Could you check a few things on this model? Use its own coordinates, in mm. A direction names the side the tool comes from. Give positions to 0.01 mm unless a question says otherwise; leave off trailing zeros. Write each loop counter-clockwise with the first axis right and the second up, starting at its lowest first coordinate (ties: lowest second). Pieces come first, ordered by that corner, then holes. Notation, with made-up numbers: M -28,-8.75 L -19,-8.75 A28 cw -19,19.25 Z; hole C 12,5 d7. An arc over 180 degrees is marked long. Use one line per item in the form item = value.
from build123d import *

# Parameters (mm, degrees)
CROQUIS1_W              = 45.25
CROQUIS1_H              = 20.4
SALIENTE_EXTRUIR1_DEPTH = 3
CROQUIS2_W              = 10.2
CROQUIS2_H              = 3
CORTAR_EXTRUIR1_DEPTH   = 50.726476851
CORTAR_EXTRUIR2_DEPTH   = 1.05
CROQUIS5_R              = 1.05
CORTAR_EXTRUIR4_DEPTH   = 50.726476851
SALIENTE_EXTRUIR2_DEPTH = 30
CROQUIS8_W              = 45.25
CROQUIS8_H              = 30
CORTAR_EXTRUIR5_DEPTH   = 10
CROQUIS10_R             = 1.65
CORTAR_EXTRUIR6_DEPTH   = 58.197574249
CROQUIS11_W             = 45.25
CROQUIS11_H             = 30
CORTAR_EXTRUIR7_DEPTH   = 2


with BuildPart() as part:
    # Croquis1 → Saliente-Extruir1 (new body)
    with BuildSketch(Plane(origin=(0, 0, 0), x_dir=(1, 0, 0), z_dir=(0, 1, 0))):
        with Locations((22.625, 10.2)):
            Rectangle(CROQUIS1_W, CROQUIS1_H)
    extrude(amount=SALIENTE_EXTRUIR1_DEPTH)

    # Croquis2 → Cortar-Extruir1 (cut, through all)
    with BuildSketch(Plane(origin=(0, 3, 0), x_dir=(1, 0, 0), z_dir=(0, 1, 0))):
        with Locations((22.625, 1.5)):
            Rectangle(CROQUIS2_W, CROQUIS2_H)
    extrude(amount=-CORTAR_EXTRUIR1_DEPTH, mode=Mode.SUBTRACT)

    # Croquis3 → Cortar-Extruir2 (cut)
    with BuildSketch(Plane(origin=(0, 3, 0), x_dir=(1, 0, 0), z_dir=(0, 1, 0))):
        Polygon((42.5, 0), (27.725, 0), (27.725, 4.51852132), (17.525, 4.51852132), (17.525, 0), (2.75, 0), (2.75, 2.75), (0, 2.75), (0, 17.65), (2.75, 17.65), (2.75, 20.4), (42.5, 20.4), (42.5, 17.65), (45.25, 17.65), (45.25, 2.75), (42.5, 2.75), align=None)
    extrude(amount=-CORTAR_EXTRUIR2_DEPTH, mode=Mode.SUBTRACT)

    # Croquis5 → Cortar-Extruir4 (cut, through all)
    with BuildSketch(Plane(origin=(0, 3, 0), x_dir=(1, 0, 0), z_dir=(0, 1, 0))):
        with Locations(Location((43.85, 18.96, 0), (0, 0, 270))):
            Circle(CROQUIS5_R)
        with Locations(Location((1.4, 18.96, 0), (0, 0, 90))):
            Circle(CROQUIS5_R)
        with Locations(Location((43.85, 1.44, 0), (0, 0, 90))):
            Circle(CROQUIS5_R)
        with Locations(Location((1.4, 1.44, 0), (0, 0, 270))):
            Circle(CROQUIS5_R)
    extrude(amount=-CORTAR_EXTRUIR4_DEPTH, mode=Mode.SUBTRACT)

    # Croquis6 → Saliente-Extruir2 (add)
    with BuildSketch(Plane.XZ):
        Polygon((17.525, -3), (0, -3), (0, -18), (45.25, -18), (45.25, -3), align=None)
    extrude(amount=SALIENTE_EXTRUIR2_DEPTH)

    # Croquis8 → Cortar-Extruir5 (cut)
    with BuildSketch(Plane.XY.offset(-3)):
        with Locations((22.625, -15)):
            Rectangle(CROQUIS8_W, CROQUIS8_H)
    extrude(amount=-CORTAR_EXTRUIR5_DEPTH, mode=Mode.SUBTRACT)

    # Croquis10 → Cortar-Extruir6 (cut, through all)
    with BuildSketch(Plane(origin=(0, 0, -18), x_dir=(-1, 0, 0), z_dir=(0, 0, -1))):
        with Locations((-11.3125, -15)):
            Circle(CROQUIS10_R)
        with Locations((-33.9375, -15)):
            Circle(CROQUIS10_R)
    extrude(amount=-CORTAR_EXTRUIR6_DEPTH, mode=Mode.SUBTRACT)

    # Croquis11 → Cortar-Extruir7 (cut)
    with BuildSketch(Plane(origin=(0, 0, -18), x_dir=(-1, 0, 0), z_dir=(0, 0, -1))):
        with Locations((-22.625, -15)):
            Rectangle(CROQUIS11_W, CROQUIS11_H)
    extrude(amount=-CORTAR_EXTRUIR7_DEPTH, mode=Mode.SUBTRACT)


solid = part.part
1) I want a section at B-B, the plane y = -15. Please give me the cut outline in (x, z).
Checked values:
outline = M 0,-16 L 9.66,-16 L 9.66,-13 L 0,-13 Z; M 12.96,-16 L 32.29,-16 L 32.29,-13 L 12.96,-13 Z; M 35.59,-16 L 45.25,-16 L 45.25,-13 L 35.59,-13 Z
2) For faces 5 (the flat face through (22.7, 2.5, -4.519)), 6 (the flat face through (42.5, 2.5, -19)), 7 (the flat face through (27.725, 2.5, -3.7)), which set-ups out of +Z, -Z, +X, -X, +Y, -Y let a thin tool reach every point of the face, with its end or its side?
Checked values:
face_5 = -Z, +X, -X, +Y
face_6 = +Z, -Z, +Y
face_7 = +Z, -Z, +X, +Y
3) Thinking about a two-plate mould opening in Z: for faces 1 (the flat face through (1.4, 2.5, -17.65)), 2 (the flat face through (17.525, 2.5, -3.8)), 3 (the flat face through (22, -15, -13)), 4 (the flat face through (1.4, 2.5, -2.75)), which applies, released by +Z, released by -Z, zero draft, split by the parting line, or undercut?
Checked values:
face_1 = undercut
face_2 = zero draft
face_3 = released by +Z
face_4 = undercut
4) I want a section at D-D, the plane z = -1.44. Please give me the cut outline in (x, y) (3 decimals), plus the area to 3 significant figures.
Checked values:
outline = M 0,0 L 0.35,0 L 0.35,3 L 0,3 Z; M 2.45,0 L 17.525,0 L 17.525,1.95 L 2.75,1.95 L 2.75,3 L 2.45,3 Z; M 27.725,0 L 42.8,0 L 42.8,3 L 42.5,3 L 42.5,1.95 L 27.725,1.95 Z; M 44.9,0 L 45.25,0 L 45.25,3 L 44.9,3 Z
area = 61.5 mm2
5) For pin 1 Ø8 at (x, y) = (18, -20.5) entering from +Z; pin 2 Ø3 at (x, z) = (30, -3) entering from -Y; pin 3 Ø5.5 at (x, y) = (11.31, -15) entering from -Z, each with a flat end and sliding along its axis, tell me the tip position at first contact or that it passes through.
Checked values:
pin_1 = -13
pin_2 = 0
pin_3 = -16
6) If I drill on L1, parallel to X at y = 1.7, z = -18.96; L2, parallel to X at y = 0.6, z = -1.44 (3 decimals); L3, parallel to Z at x = 43, y = 1, over which ranges is the centre line in solid material (lowest first)?
Checked values:
L1 = 0 to 0.35, 2.45 to 42.8, 44.9 to 45.25
L2 = 0 to 0.35, 2.45 to 17.525, 27.725 to 42.8, 44.9 to 45.25
L3 = -20.4 to -19.58, -18.34 to -2.06, -0.82 to 0
7) I want a section at A-A, the plane x = 43.85. Please give me the cut outline in (y, z), plus the area to 3 significant figures.
Checked values:
outline = M -30,-16 L 0,-16 L 0,-17.91 L 3,-17.91 L 3,-17.65 L 1.95,-17.65 L 1.95,-2.75 L 3,-2.75 L 3,-2.49 L 0,-2.49 L 0,-13 L -30,-13 Z; M 0,-20.4 L 3,-20.4 L 3,-20.01 L 0,-20.01 Z; M 0,-0.39 L 3,-0.39 L 3,0 L 0,0 Z
area = 123 mm2
8) I want a section at C-C, the plane z = -18.96. Please give me the cut outline in (x, y).
Checked values:
outline = M 0,0 L 0.35,0 L 0.35,3 L 0,3 Z; M 2.45,0 L 42.8,0 L 42.8,3 L 42.5,3 L 42.5,1.95 L 2.75,1.95 L 2.75,3 L 2.45,3 Z; M 44.9,0 L 45.25,0 L 45.25,3 L 44.9,3 Z
